```python
from build123d import *

# Parameters (mm, degrees)
SKETCH1_W           = 45
SKETCH1_H           = 30
BOSS_EXTRUDE1_DEPTH = 2
SKETCH2_R           = 9
SKETCH2_R_2         = 6
CUT_EXTRUDE1_DEPTH  = 20
SKETCH3_W           = 2
SKETCH3_H           = 30
BOSS_EXTRUDE2_DEPTH = 70
CHAMFER1_SIZE       = 10


with BuildPart() as part:
    # Sketch1 → Boss-Extrude1 (new body)
    with BuildSketch(Plane(origin=(0, 0, 0), x_dir=(1, 0, 0), z_dir=(0, 1, 0))):
        with Locations((22.5, 15)):
            Rectangle(SKETCH1_W, SKETCH1_H)
    extrude(amount=BOSS_EXTRUDE1_DEPTH)

    # Sketch2 → Cut-Extrude1 (cut)
    with BuildSketch(Plane(origin=(0, 2, 0), x_dir=(1, 0, 0), z_dir=(0, 1, 0))):
        with Locations((10, 15)):
            Circle(SKETCH2_R)
        with Locations((30, 15)):
            Circle(SKETCH2_R_2)
    extrude(amount=-CUT_EXTRUDE1_DEPTH, mode=Mode.SUBTRACT)

    # Sketch3 → Boss-Extrude2 (add)
    with BuildSketch(Plane.XZ):
        with Locations((44, -15)):
            Rectangle(SKETCH3_W, SKETCH3_H)
    extrude(amount=BOSS_EXTRUDE2_DEPTH)

    # Chamfer1
    chamfer1_edges = [part.edges().sort_by_distance(p)[0] for p in [
        (0, 1, -30),
    ]]
    chamfer(chamfer1_edges, length=CHAMFER1_SIZE)


solid = part.part
```
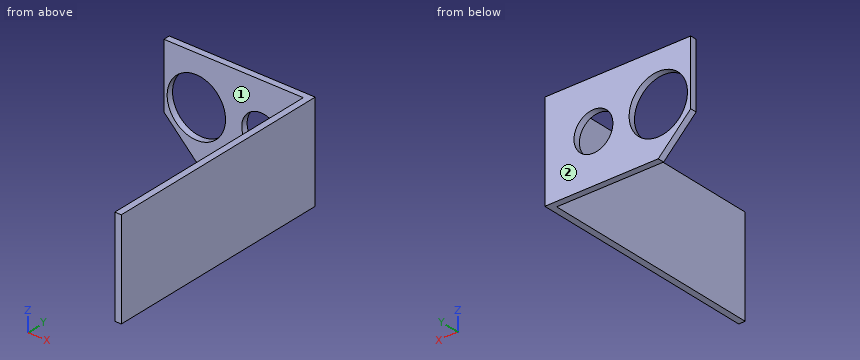
For this review, take the finished solid that the model builds, in its own axes (mm). Face numbers are marked on the shaded views. A direction names the side the tool comes from. Coordinates: 2 decimals unless noted, no trailing zeros. Loops run counter-clockwise (first coordinate to the right, second up) from the corner with the lowest first, then second, coordinate; pieces in that order, holes last.
1. For the marked faces 1 and 2, list the 3-axis set-ups (+Z, -Z, +X, -X, +Y, -Y) from which the entire face can be reached by the end or side of a thin tool; tool diameter is ignored.
2. Add section A-A, the plane x = 30. Give the boundary of the cut face in (y, z).
3. Add section D-D, the plane x = 25.5. Give the boundary of the cut face in (y, z).
4. For line 1 (X direction, y = 1.4, z = -15); line 2 (Z direction, x = 10, y = 0.45); line 3 (Y direction, x = 32, z = -22.75), list the stretches that pass through material, from the lowest coordinate up.
5. Insertion check: P1, Ø15, axis at x = 20, z = -22, coming from the -Y side; P2, Ø16, axis at x = 10, z = -15, coming from the +Y side; P3, Ø15, axis at y = -35, z = -13, coming from the -X side. Each pin has a flat end and moves straight along its axis. Give the tip position at first contact, or say it passes through.
6. Add section B-B, the plane z = -15. Give the boundary of the cut face in (x, y), then the cut area to 3 significant figures.
7. Add section C-C, the plane z = -3. Give the boundary of the cut face in (x, y), then the cut area to 3 significant figures.
Result:
1. face 1: +Z, -Z, -X, -Y
1. face 2: +Z, -Z, +X, -X, +Y
2. outline: (0, -30) - (2, -30) - (2, -21) - (0, -21) - close; (0, -9) - (2, -9) - (2, 0) - (0, 0) - close
3. outline: (0, -30) - (2, -30) - (2, -18.97) - (0, -18.97) - close; (0, -11.03) - (2, -11.03) - (2, 0) - (0, 0) - close
4. line 1: x = 0 to 1, 19 to 24, 36 to 45
4. line 2: z = -30 to -24, -6 to 0
4. line 3: y = 0 to 2
5. P1: stops at y = 0
5. P2: passes through
5. P3: stops at x = 43
6. outline: (0, 0) - (1, 0) - (1, 2) - (0, 2) - close; (19, 0) - (24, 0) - (24, 2) - (19, 2) - close; (36, 0) - (43, 0) - (43, -70) - (45, -70) - (45, 2) - (36, 2) - close
6. area: 170 mm2
7. outline: (0, 0) - (43, 0) - (43, -70) - (45, -70) - (45, 2) - (0, 2) - close
7. area: 230 mm2
